Here's how the part is built. I have some questions about the finished solid (model axes, mm). A direction names the side the tool comes from. Give positions to 0.01 mm unless a question says otherwise; leave off trailing zeros. Order: outer loops, then holes, each group sorted by start corner. A loop starts at its lowest first (then second) coordinate and runs counter-clockwise, first axis right, second up. Notation, with made-up numbers: M 50,-10 L 97,-10 A14 ccw 97,6 Z; hole C -7.75,-1.75 d10. An arc over 180 degrees is marked long. Use CSV: the item, a comma, the result in double quotes. Start each with the question number.
```python
from build123d import *

# Parameters (mm, degrees)
PAD005_DEPTH = 180
PAD004_DEPTH = 10
PAD002_DEPTH = 15
PAD003_DEPTH = 10
PAD001_DEPTH = 15
PAD_DEPTH    = 150
CHAMFER_SIZE = 1.9


with BuildPart() as body005:
    # Sketch005 → Pad005 (new body)
    with BuildSketch(Plane.XY):
        Polygon((0, 23), (23, 16.837169), (23, -16.837169), (0, -23), (-23, -16.837169), (-23, 16.837169), align=None)
    extrude(amount=PAD005_DEPTH)


with BuildPart() as body004:
    # Sketch004 → Pad004 (new body)
    with BuildSketch(Plane.XY):
        Polygon((0, 25.25), (25.25, 18.484283), (25.25, -18.484283), (0, -25.25), (-25.25, -18.484283), (-25.25, 18.484283), align=None)
    extrude(amount=PAD004_DEPTH)


with BuildPart() as body004_1:
    # Body004 placement: moved
    add(body004.part.moved(Location((0, 0, 5))))


with BuildPart() as cut001:
    # Sketch002 → Pad002 (new body)
    with BuildSketch(Plane.XY):
        Polygon((0, 27.5), (27.5, 20.131397), (27.5, -20.131397), (0, -27.5), (-27.5, -20.131397), (-27.5, 20.131397), align=None)
    extrude(amount=PAD002_DEPTH)

    # Cut001: cut Body004
    add(body004_1.part, mode=Mode.SUBTRACT)


with BuildPart() as cut001_1:
    # Cut001 placement: moved
    add(cut001.part.moved(Location((0, 0, 165))))


with BuildPart() as body003:
    # Sketch003 → Pad003 (new body)
    with BuildSketch(Plane.XY):
        Polygon((0, 25.25), (25.25, 18.484283), (25.25, -18.484283), (0, -25.25), (-25.25, -18.484283), (-25.25, 18.484283), align=None)
    extrude(amount=PAD003_DEPTH)


with BuildPart() as cut:
    # Sketch001 → Pad001 (new body)
    with BuildSketch(Plane.XY):
        Polygon((0, 27.5), (27.5, 20.131397), (27.5, -20.131397), (0, -27.5), (-27.5, -20.131397), (-27.5, 20.131397), align=None)
    extrude(amount=PAD001_DEPTH)

    # Cut: cut Body003
    add(body003.part, mode=Mode.SUBTRACT)


with BuildPart() as chamfer_body:
    # Sketch → Pad (new body)
    with BuildSketch(Plane.XY):
        Polygon((0, 25), (25, 18.30127), (25, -18.30127), (0, -25), (-25, -18.30127), (-25, 18.30127), align=None)
    extrude(amount=PAD_DEPTH)


with BuildPart() as chamfer_body_1:
    # Body placement: moved
    add(chamfer_body.part.moved(Location((0, 0, 15))))

    # Fusion: union Cut
    add(cut.part)

    # Fusion001: union Cut001
    add(cut001_1.part)

    # Cut002: cut Body005
    add(body005.part, mode=Mode.SUBTRACT)

    # Chamfer
    chamfer_edges = [chamfer_body_1.edges().sort_by_distance(p)[0] for p in [
        (-25, 0, 165),
        (-12.5, -21.650635, 165),
        (12.5, -21.650635, 165),
        (25, 0, 165),
        (12.5, 21.650635, 165),
        (-12.5, 21.650635, 165),
        (-25, 0, 15),
        (-12.5, -21.650635, 15),
        (12.5, -21.650635, 15),
        (25, 0, 15),
        (12.5, 21.650635, 15),
        (-12.5, 21.650635, 15),
    ]]
    chamfer(chamfer_edges, length=CHAMFER_SIZE)


solid = chamfer_body_1.part
```
Q1. Imagine slicing it at A-A, the plane y = -6.5. Please give me the cut outline in (x, z).
Q2. I need wall thicknesses on line 1 (X direction, y = -10, z = 118); line 2 (Z direction, x = -12, y = -24); line 3 (Y direction, x = -0.5, z = 171). Which ranges of each line are inside material? Lowest first, please. Write a range as [from, to].
Q3. For faces 1 (the face through (-12.325, -21.698, 88.977)), 2 (the face through (12.448, 21.915, 174.93)), 3 (the face through (3.9, -22.3, 10)), 4 (the face through (-12.675, 21.604, 88.977)), which set-ups out of +Z, -Z, +X, -X, +Y, -Y let a thin tool reach every point of the face, with its end or its side?
Q4. For P1, Ø2, axis at x = -5.5, z = 106.5, coming from the +Y side; P2, Ø10, axis at y = -7.5, z = 91, coming from the +X side; P3, Ø3, axis at x = 21.5, z = 52, coming from the -Y side, each with a flat end and sliding along its axis, tell me the tip position at first contact or that it passes through.
Q5. Imagine slicing it at B-B, the plane z = 62. Please give me the cut outline in (x, y), then the cut area to 3 significant figures.
Q6. We'd pull the mould along X, two halves only. Please class faces 5 (the face through (12.8, -21.82, 174.93)), 6 (the face through (-13.942, 23.764, 172.395)), 7 (the face through (10.31, 24.57, 165)): pulls with the +X half, pulls with the -X half, needs draft (parallel to the pull), parting line crosses it, or undercut.
Q7. Imagine slicing it at C-C, the plane x = -18. Please give me the cut outline in (y, z), then the cut area to 3 significant figures.
Reply:
1,outline,"M -27.5,0 L -25.25,0 L -25.25,10 L -23,10 L -23,170 L -25.25,170 L -25.25,180 L -27.5,180 L -27.5,165 L -26.9,165 L -25,163.1 L -25,16.9 L -26.9,15 L -27.5,15 Z; M 23,10 L 25.25,10 L 25.25,0 L 27.5,0 L 27.5,15 L 26.9,15 L 25,16.9 L 25,163.1 L 26.9,165 L 27.5,165 L 27.5,180 L 25.25,180 L 25.25,170 L 23,170 Z"
2,line 1,"x = [-25, -23], [23, 25]"
2,line 2,"z = [0, 15], [165, 180]"
2,line 3,"y = [-27.37, -25.12], [25.12, 27.37]"
3,face 1,"-X, -Y"
3,face 2,"+Z"
3,face 3,"-Z"
3,face 4,"-X, +Y"
4,P1,"stops at y = 23.79"
4,P2,"stops at x = 25"
4,P3,"stops at y = -19.64"
5,outline,"M -25,-18.3 L 0,-25 L 25,-18.3 L 25,18.3 L 0,25 L -25,18.3 Z; hole M -23,-16.84 L 0,-23 L 23,-16.84 L 23,16.84 L 0,23 L -23,16.84 Z"
5,area,"333 mm^2"
6,face 5,"undercut"
6,face 6,"pulls with the -X half"
6,face 7,"needs draft"
7,outline,"M -22.68,0 L -20.43,0 L -20.43,10 L -18.18,10 L -18.18,170 L -20.43,170 L -20.43,180 L -22.68,180 L -22.68,165 L -22.14,165 L -20.18,163.1 L -20.18,16.9 L -22.14,15 L -22.68,15 Z; M 18.18,10 L 20.43,10 L 20.43,0 L 22.68,0 L 22.68,15 L 22.14,15 L 20.18,16.9 L 20.18,163.1 L 22.14,165 L 22.68,165 L 22.68,180 L 20.43,180 L 20.43,170 L 18.18,170 Z"
7,area,"787 mm^2"
